Part print with two shaded views. Sizes in mm from the minimum x, y, z corner. Give positions to 0.01 mm unless a question says otherwise; leave off trailing zeros. Write each loop counter-clockwise with the first axis right and the second up, starting at its lowest first coordinate (ties: lowest second). Pieces come first, ordered by that corner, then holes. Notation, with made-up numbers: (49, 85.25) -> (71, 85.25) arc R11 ccw to (71, 94.25) -> close; hole circle Ø9 at (19, 37.5). An arc over 180 degrees is marked (long way). Answer in a Markdown table with one row per item. Add a question column.
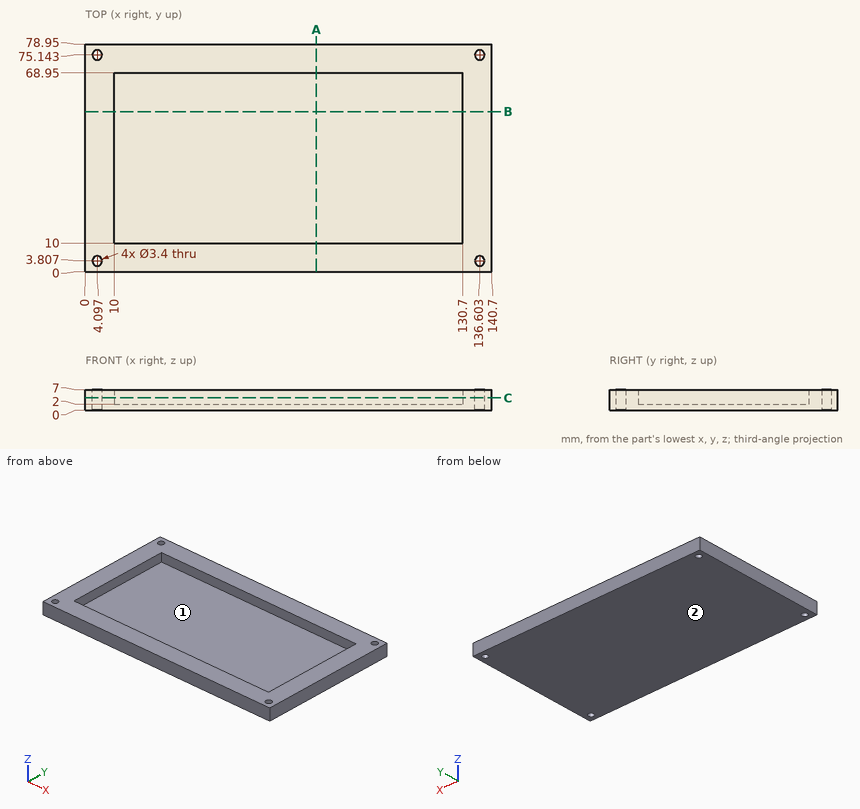
Item 1: Drop flat-ended pins along their axis: pin 1 Ø3 at (x, y) = (89, 29.5) entering from -Z; pin 2 Ø8 at (x, y) = (89.5, 53) entering from +Z. Give the stop position or say it passes through.
Item 2: Slice it at B-B, the plane y = 55.5. List the corners of the cut face in (x, z).
Item 3: Probe L1, parallel to Y at x = 55, z = 3; L2, parallel to X at y = 20.5, z = 5; L3, parallel to X at y = 74, z = 5.25 (1 decimal). List the from-to ranges inside material, lowest first. Write a range as from..to.
Item 4: Mould opens along Y. For the marked faces 1 and 2 say: released by +Y, released by -Y, zero draft, split by the parting line, or undercut.
Item 5: Slice it at A-A, the plane x = 80. List the corners of the cut face in (y, z), then the cut area to 3 significant figures.
Item 6: Slice it at C-C, the plane z = 4.25. List the corners of the cut face in (x, y), then the cut area to 3 significant figures.
Answer key:
| question | item | result |
|---|---|---|
| 1 | pin 1 | stops at z = 0 |
| 1 | pin 2 | stops at z = 2 |
| 2 | outline | (0, 0) -> (140.7, 0) -> (140.7, 7) -> (130.7, 7) -> (130.7, 2) -> (10, 2) -> (10, 7) -> (0, 7) -> close |
| 3 | L1 | y = 0..10, 68.95..78.95 |
| 3 | L2 | x = 0..10, 130.7..140.7 |
| 3 | L3 | x = 0..2.8, 5.4..135.3, 137.9..140.7 |
| 4 | face 1 | undercut |
| 4 | face 2 | zero draft |
| 5 | outline | (0, 0) -> (78.95, 0) -> (78.95, 7) -> (68.95, 7) -> (68.95, 2) -> (10, 2) -> (10, 7) -> (0, 7) -> close |
| 5 | area | 258 mm² |
| 6 | outline | (0, 0) -> (140.7, 0) -> (140.7, 78.95) -> (0, 78.95) -> close; hole circle Ø3.4 at (4.1, 3.81); hole circle Ø3.4 at (4.1, 75.14); hole (10, 10) -> (130.7, 10) -> (130.7, 68.95) -> (10, 68.95) -> close; hole circle Ø3.4 at (136.6, 3.81); hole circle Ø3.4 at (136.6, 75.14) |
| 6 | area | 3,960 mm² |
